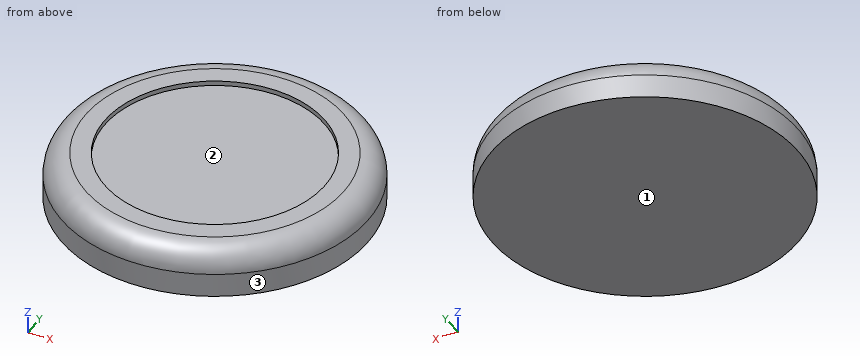
```python
from build123d import *

# Parameters (mm, degrees)
F0_R     = 16
F1_DEPTH = 5
F2_T     = -4.5
F3_R     = 2.5


with BuildPart() as f1:
    # F0 (on Top) → F1 (new body)
    with BuildSketch(Plane.XY):
        with Locations((-13.779012, 0)):
            Circle(F0_R)
    extrude(amount=F1_DEPTH)

    # F2
    f2_openings = [f1.faces().sort_by_distance(p)[0] for p in [
        (-13.779012, 0, 5),
    ]]
    offset(amount=F2_T, openings=f2_openings)

    # F3
    f3_edges = [f1.edges().sort_by_distance(p)[0] for p in [
        (-29.779012, 0, 5),
    ]]
    fillet(f3_edges, radius=F3_R)


solid = f1.part
```
Design review of the part built by this model. Coordinates are the model's own, in mm. Face numbers are marked on the shaded views. Coordinates: 2 decimals unless noted, no trailing zeros. Order: outer loops, then holes, each group sorted by start corner. A loop starts at its lowest first (then second) coordinate and runs counter-clockwise, first axis right, second up.
1) Wall thickness on line 1 along Z through (x, y) = (-24, 0.5); line 2 along Z through (x, y) = (-5, 10.5); line 3 along X through (y, z) = (14, 0.6): over which ranges is each line inside the solid? List them lowest first.
2) Mouldability with a two-part tool opening along X and no side actions: class the marked faces 1, 2 and 3 as +X half, -X half, draft (parallel to the pull), parting line (faces both ways), or undercut.
3) Clearance check with flat-ended pins moving along their axes: pin 1 (3 mm diameter, centred on y = -9.5, z = 2.5, fed in from -X); pin 2 (7 mm diameter, centred on x = -19, y = -2.5, fed in from +Z); pin 3 (1.5 mm diameter, centred on y = -5, z = 4, fed in from +X). State where each tip first meets the part, or that it passes through.
4) Take a section at C-C, the plane z = 4. Give the boundary of the cut face in (x, y), and give its area (3 significant figures).
5) Take a section at A-A, the plane y = 0. Give the boundary of the cut face in (x, z), and give its area (3 significant figures).
6) Take a section at B-B, the plane z = 1.75. Give the boundary of the cut face in (x, y).
Returned:
1. line 1: z = 0 to 4.5
1. line 2: z = 0 to 4.99
1. line 3: x = -21.52 to -6.03
2. face 1: draft
2. face 2: undercut
2. face 3: parting line
3. pin 1: stops at x = -27.64
3. pin 2: stops at z = 4.5
3. pin 3: stops at x = 1.39
4. outline: circle Ø31 at (-13.78, 0)
4. area: 755 mm2
5. outline: (-29.78, 0) - (2.22, 0) - (2.22, 2.5) arc R2.5 ccw to (-0.28, 5) - (-2.28, 5) - (-2.28, 4.5) - (-25.28, 4.5) - (-25.28, 5) - (-27.28, 5) arc R2.5 ccw to (-29.78, 2.5) - close
5. area: 146 mm2
6. outline: circle Ø32 at (-13.78, 0)
